Here's the drawing with two shaded views (mm, measured from the low corner). I have some questions. Coordinates: 2 decimals unless noted, no trailing zeros. Write each loop counter-clockwise with the first axis right and the second up, starting at its lowest first coordinate (ties: lowest second). Pieces come first, ordered by that corner, then holes. Notation, with made-up numbers: (7, -37.5) -> (17, -37.5) arc R23 ccw to (17, -14.5) -> close; hole circle Ø5 at (39.25, 7.5). An arc over 180 degrees is marked (long way). Answer in a Markdown table with one row per item. Add a question column.
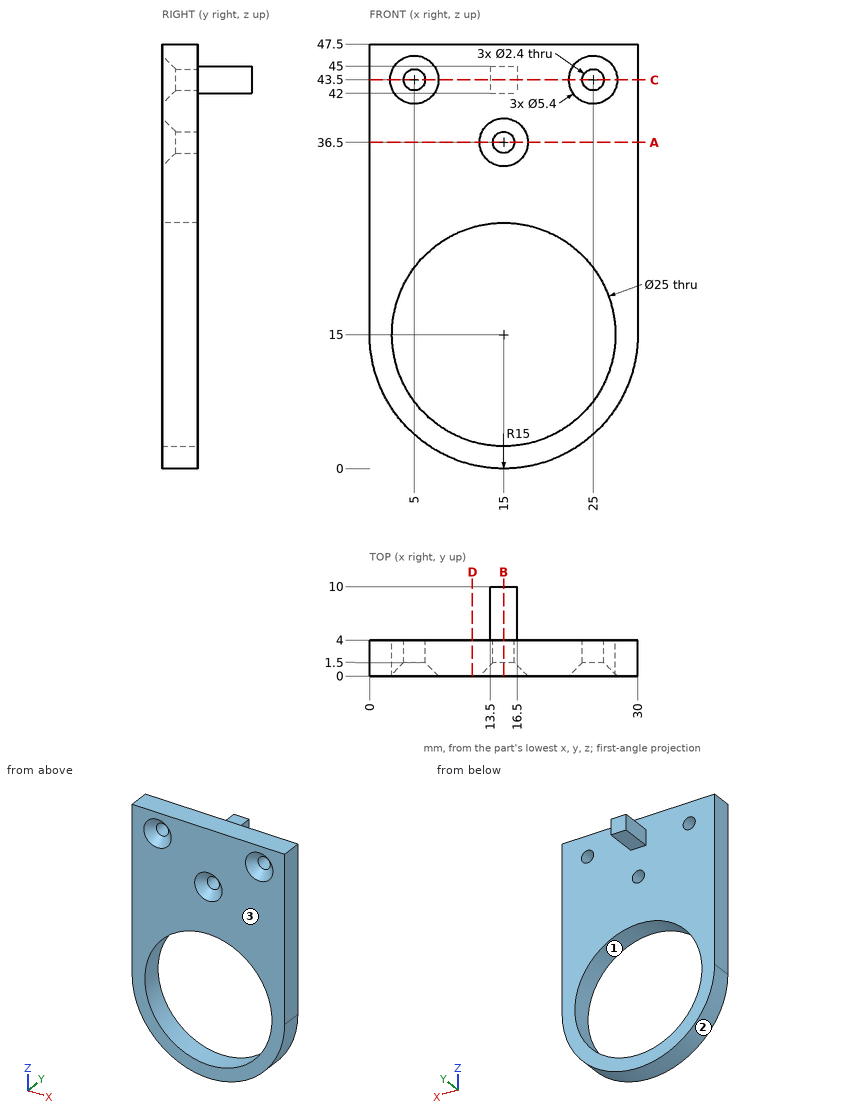
Q1. I need wall thicknesses on line 1 (X direction, y = 2.95, z = 43.5); line 2 (X direction, y = 3, z = 15); line 3 (X direction, y = 0.75, z = 44). Which ranges of each line are inside material? Lowest first, please. Write a range as [from, to].
Q2. I'm going to push flat-ended pins straight in: P1, Ø5, axis at x = 13, z = 28.5, coming from the +Y side; P2, Ø3, axis at x = 15, z = 36.5, coming from the -Y side; P3, Ø9, axis at x = 12.5, z = 21.5, coming from the +Y side; P4, Ø1.5, axis at x = 14.5, y = 6, coming from the +Z side. Where does each tip first touch, or does it pass through?
Q3. Imagine slicing it at C-C on z = 43.5. Please give me the cut outline in (x, y).
Q4. Imagine slicing it at A-A on z = 36.5. Please give me the cut outline in (x, y), plus the area to 3 significant figures.
Q5. Imagine slicing it at B-B on x = 15. Please give me the cut outline in (y, z), plus the area to 4 significant figures.
Q6. Imagine slicing it at D-D on x = 11.5. Please give me the cut outline in (y, z).
Q7. If we mould it in two halves opening along X, with no side actions, what happens to the marked faces 1, 2 and 3? For each: pulls with the +X half, pulls with the -X half, needs draft (parallel to the pull), parting line crosses it, or undercut.
Result sheet:
| question | item | result |
|---|---|---|
| 1 | line 1 | x = [0, 3.8], [6.2, 23.8], [26.2, 30] |
| 1 | line 2 | x = [0, 2.5], [27.5, 30] |
| 1 | line 3 | x = [0, 3.12], [6.88, 23.12], [26.88, 30] |
| 2 | P1 | stops at y = 4 |
| 2 | P2 | stops at y = 1.2 |
| 2 | P3 | passes through |
| 2 | P4 | stops at z = 45 |
| 3 | outline | (0, 0) -> (2.3, 0) -> (3.8, 1.5) -> (3.8, 4) -> (0, 4) -> close; (6.2, 1.5) -> (7.7, 0) -> (22.3, 0) -> (23.8, 1.5) -> (23.8, 4) -> (16.5, 4) -> (16.5, 10) -> (13.5, 10) -> (13.5, 4) -> (6.2, 4) -> close; (26.2, 1.5) -> (27.7, 0) -> (30, 0) -> (30, 4) -> (26.2, 4) -> close |
| 4 | outline | (0, 0) -> (12.3, 0) -> (13.8, 1.5) -> (13.8, 4) -> (0, 4) -> close; (16.2, 1.5) -> (17.7, 0) -> (30, 0) -> (30, 4) -> (16.2, 4) -> close |
| 4 | area | 108 mm^2 |
| 5 | outline | (0, 0) -> (4, 0) -> (4, 2.5) -> (0, 2.5) -> close; (0, 27.5) -> (4, 27.5) -> (4, 35.3) -> (1.5, 35.3) -> (0, 33.8) -> close; (0, 39.2) -> (1.5, 37.7) -> (4, 37.7) -> (4, 42) -> (10, 42) -> (10, 45) -> (4, 45) -> (4, 47.5) -> (0, 47.5) -> close |
| 5 | area | 96.15 mm^2 |
| 6 | outline | (0, 0.41) -> (4, 0.41) -> (4, 3) -> (0, 3) -> close; (0, 27) -> (4, 27) -> (4, 47.5) -> (0, 47.5) -> close |
| 7 | face 1 | undercut |
| 7 | face 2 | parting line crosses it |
| 7 | face 3 | needs draft |
